The model under review builds one solid part; all positions refer to its coordinate system, in mm. Face numbers are marked on the shaded views. A direction names the side the tool comes from. Round coordinates to 2 decimals unless told otherwise and drop trailing zeros. Loops run counter-clockwise (first coordinate to the right, second up) from the corner with the lowest first, then second, coordinate; pieces in that order, holes last. Notation, with made-up numbers: M 65,9.25 L 113,9.25 A29 ccw 113,45.25 Z; hole C -18.75,57.25 d11. An arc over 180 degrees is marked long. Answer as a JSON object with one key per item and string values. Group by question number.
Item 1: The part is to be moulded in two halves that separate along X. For the marked faces 3 and 4, say which applies: +X half, -X half, draft (parallel to the pull), parting line (faces both ways), or undercut.
Item 2: Tool access review of the marked faces 1 and 2: name each direction out of +Z, -Z, +X, -X, +Y, -Y from which nothing blocks a thin tool from reaching the whole face with its end or side.
Item 3: Insertion check: P1, Ø2, axis at x = -8.5, z = -18, coming from the +Y side; P2, Ø2, axis at x = 1.5, z = 13.5, coming from the -Y side; P3, Ø5, axis at x = 14, y = -11.5, coming from the +Z side; P4, Ø3, axis at x = -1.5, y = 7.5, coming from the +Z side. Each pin has a flat end and moves straight along its axis. Give the tip position at first contact, or say it passes through.
Item 4: To check wall thickness, follow line 1 (X direction, y = 0, z = 15.75); line 2 (Y direction, x = 0, z = -23). State the ranges of each line that lie inside material, in increasing order.
Item 5: Consider section A-A (z = 17.5). Give the boundary of the cut face in (x, y).
```python
from build123d import *

# Parameters (mm, degrees)
FILLET_R    = 8
FILLET001_R = 8
FILLET002_R = 2
FILLET003_R = 2


with BuildPart() as part:
    # Sketch → Revolution (revolve)
    with BuildSketch(Plane.XZ):
        Polygon((-11.22, 21.8), (-11.22, 1.8), (-20, 1.8), (-20, -28), (-18.2, -28), (-18.2, 0), (-9.42, 0), (-9.42, 21.8), align=None)
    revolve(axis=Axis((0, 0, 0), (0, 0, 1)))

    # Fillet
    fillet_edges = [part.edges().sort_by_distance(p)[0] for p in [
        (18.2, 0, 0),
    ]]
    fillet(fillet_edges, radius=FILLET_R)

    # Fillet001
    fillet001_edges = [part.edges().sort_by_distance(p)[0] for p in [
        (20, 0, 1.8),
    ]]
    fillet(fillet001_edges, radius=FILLET001_R)

    # Fillet002
    fillet002_edges = [part.edges().sort_by_distance(p)[0] for p in [
        (11.22, 0, 1.8),
    ]]
    fillet(fillet002_edges, radius=FILLET002_R)

    # Fillet003
    fillet003_edges = [part.edges().sort_by_distance(p)[0] for p in [
        (9.42, 0, 0),
    ]]
    fillet(fillet003_edges, radius=FILLET003_R)


solid = part.part
```
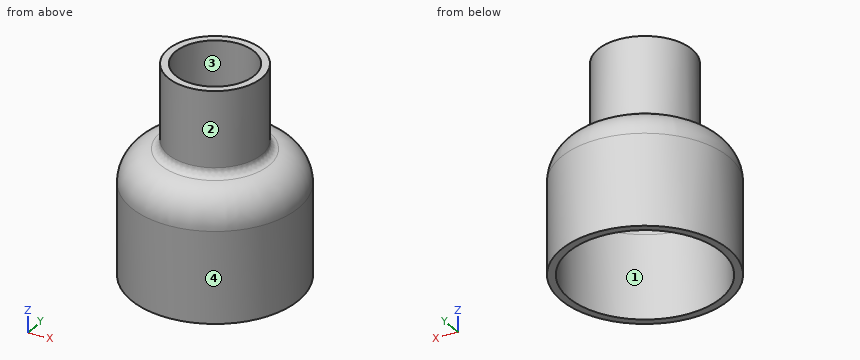
Geometry results:
{
 "1": {"face 3": "undercut", "face 4": "parting line"},
 "2": {"face 1": "-Z", "face 2": "+Z"},
 "3": {"P1": "stops at y = 18.54", "P2": "stops at y = -11.21", "P3": "stops at z = 0.94", "P4": "passes through"},
 "4": {"line 1": "x = -11.22 to -9.42, 9.42 to 11.22", "line 2": "y = -20 to -18.2, 18.2 to 20"},
 "5": {"outline": "C 0,0 d22.44; hole C 0,0 d18.84"}
}
